from build123d import *

# Parameters (mm, degrees)
BOSS_EXTRUDE1_DEPTH = 14
SKETCH2_R           = 4
CUT_EXTRUDE1_DEPTH  = 11


with BuildPart() as part:
    # Sketch1 → Boss-Extrude1 (new body)
    with BuildSketch(Plane.XY):
        with BuildLine():
            Line((-8.817662135, -6.081589164), (16.182337865, -6.081589164))
            Line((16.182337865, -6.081589164), (16.182337865, 3.918410836))
            Line((16.182337865, 3.918410836), (22.182337865, 3.918410836))
            Line((22.182337865, 3.918410836), (22.182337865, 6.418410836))
            Line((22.182337865, 6.418410836), (2.079389137, 6.418410836))
            ThreePointArc((2.079389137, 6.418410836), (-6.21204118, 2.646753081), (-8.817662135, -6.081589164))
        make_face()
    extrude(amount=BOSS_EXTRUDE1_DEPTH)

    # Sketch2 → Cut-Extrude1 (cut)
    with BuildSketch(Plane.XZ.offset(6.081589164)):
        with Locations(Location((7.905122548, 7, 0), (0, 0, 270))):
            Circle(SKETCH2_R)
    extrude(amount=-CUT_EXTRUDE1_DEPTH, mode=Mode.SUBTRACT)


solid = part.part
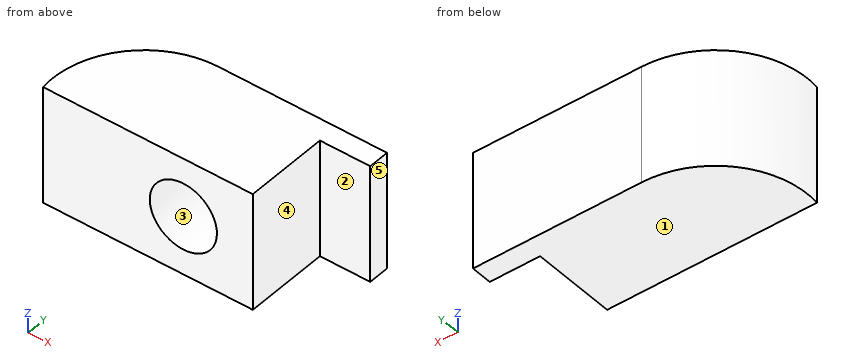
Geometry: final body of the model. Coordinates: model frame, mm. Face numbers are marked on the shaded views. A direction names the side the tool comes from. Coordinates: 2 decimals unless noted, no trailing zeros. Write each loop counter-clockwise with the first axis right and the second up, starting at its lowest first coordinate (ties: lowest second). Pieces come first, ordered by that corner, then holes. Notation, with made-up numbers: (40, 38.25) - (86, 38.25) arc R32 ccw to (86, 74.25) - close; hole circle Ø10 at (85, 23.5). An arc over 180 degrees is marked (long way). Return JSON: item names as keys, results as strings.
Item 1: Pull-direction query (Z, two-part tool) for the marked faces 1, 2 and 3; classes: +Z half, -Z half, draft (parallel to the pull), parting line (faces both ways), or undercut.
Completed:
{"face 1": "-Z half", "face 2": "draft", "face 3": "undercut"}
Item 2: Pin query (flat end, axial travel): pin 1 Ø5 at (y, z) = (-1, 12) entering from -X; pin 2 Ø4 at (x, z) = (6.5, 7.5) entering from -Y; pin 3 Ø3 at (x, z) = (19.5, 5.5) entering from -Y. Return the tip coordinate at first contact, or that it passes through.
Completed:
{"pin 1": "stops at x = -8.87", "pin 2": "stops at y = 4.92", "pin 3": "stops at y = 3.92"}
Item 3: Section query C-C (x = 10.5). Output: boundary loops of the cut face in (y, z).
Completed:
{"outline": "(-6.08, 0) - (6.42, 0) - (6.42, 14) - (-6.08, 14) - (-6.08, 10.04) - (4.92, 10.04) - (4.92, 3.96) - (-6.08, 3.96) - close"}
Item 4: Section query D-D (z = 4.75). Output: boundary loops of the cut face in (x, y), and give its area (3 significant figures).
Completed:
{"outline": "(-8.82, -6.08) - (4.6, -6.08) - (4.6, 4.92) - (11.21, 4.92) - (11.21, -6.08) - (16.18, -6.08) - (16.18, 3.92) - (22.18, 3.92) - (22.18, 6.42) - (2.08, 6.42) arc R11 ccw to start", "area": "230 mm2"}
Item 5: Line query: L1, parallel to Y at x = 4, z = 7.25; L2, parallel to X at y = 0.75, z = 7; L3, parallel to Y at x = 21.5, z = 4.5. Output: solid intervals per line, ascending.
Completed:
{"L1": "y = 4.92 to 6.42", "L2": "x = -7.54 to 3.91, 11.91 to 16.18", "L3": "y = 3.92 to 6.42"}
Item 6: Reachability of the marked faces 4 and 5 from +Z, -Z, +X, -X, +Y, -Y: full face, straight path, thin tool, end or side. Return the list, or none.
Completed:
{"face 4": "+Z, -Z, +X, -Y", "face 5": "+Z, -Z, +X, +Y, -Y"}
Item 7: Section query B-B (y = -4.75). Output: boundary loops of the cut face in (x, z), and give its area (3 significant figures).
Completed:
{"outline": "(-8.92, 0) - (16.18, 0) - (16.18, 14) - (-8.92, 14) - close; hole circle Ø8 at (7.91, 7)", "area": "301 mm2"}
Item 8: Section query A-A (z = 7). Output: boundary loops of the cut face in (x, y).
Completed:
{"outline": "(-8.82, -6.08) - (3.91, -6.08) - (3.91, 4.92) - (11.91, 4.92) - (11.91, -6.08) - (16.18, -6.08) - (16.18, 3.92) - (22.18, 3.92) - (22.18, 6.42) - (2.08, 6.42) arc R11 ccw to start"}
